```python
from build123d import *

# Parameters (mm, degrees)
F0_R     = 4.677056
F1_DEPTH = 5


with BuildPart() as f1:
    # F0 (on Front) → F1 (new body)
    with BuildSketch(Plane.XZ):
        with BuildLine():
            ThreePointArc((8.500315, 5.267318), (9.510565, 3.09017), (9.972951, 0.73501))
            ThreePointArc((9.972951, 0.73501), (12.080664, 2.122816), (13.312307, 4.325431))
            ThreePointArc((13.312307, 4.325431), (11.021222, 5.383442), (8.500315, 5.267318))
        make_face()
        with BuildLine():
            ThreePointArc((3.780847, 9.25771), (5.877853, 8.09017), (7.636259, 6.456589))
            ThreePointArc((7.636259, 6.456589), (8.525703, 8.81823), (8.227458, 11.324125))
            ThreePointArc((8.227458, 11.324125), (5.752048, 10.833408), (3.780847, 9.25771))
        make_face()
        with BuildLine():
            ThreePointArc((-2.382776, 9.711971), (0, 10), (2.382776, 9.711971))
            ThreePointArc((2.382776, 9.711971), (1.714213, 12.145381), (0, 13.997388))
            ThreePointArc((0, 13.997388), (-1.714213, 12.145381), (-2.382776, 9.711971))
        make_face()
        with BuildLine():
            ThreePointArc((-7.636259, 6.456589), (-5.877853, 8.09017), (-3.780847, 9.25771))
            ThreePointArc((-3.780847, 9.25771), (-5.752048, 10.833408), (-8.227458, 11.324125))
            ThreePointArc((-8.227458, 11.324125), (-8.525703, 8.81823), (-7.636259, 6.456589))
        make_face()
        with BuildLine():
            ThreePointArc((-9.972951, 0.73501), (-9.510565, 3.09017), (-8.500315, 5.267318))
            ThreePointArc((-8.500315, 5.267318), (-11.021222, 5.383442), (-13.312307, 4.325431))
            ThreePointArc((-13.312307, 4.325431), (-12.080664, 2.122816), (-9.972951, 0.73501))
        make_face()
        with BuildLine():
            ThreePointArc((-13.312307, -4.325431), (-11.021222, -5.383442), (-8.500315, -5.267318))
            ThreePointArc((-8.500315, -5.267318), (-9.510565, -3.09017), (-9.972951, -0.73501))
            ThreePointArc((-9.972951, -0.73501), (-12.080664, -2.122816), (-13.312307, -4.325431))
        make_face()
        with BuildLine():
            ThreePointArc((-8.227458, -11.324125), (-5.752048, -10.833408), (-3.780847, -9.25771))
            ThreePointArc((-3.780847, -9.25771), (-5.877853, -8.09017), (-7.636259, -6.456589))
            ThreePointArc((-7.636259, -6.456589), (-8.525703, -8.81823), (-8.227458, -11.324125))
        make_face()
        with BuildLine():
            ThreePointArc((0, -13.997388), (1.714213, -12.145381), (2.382776, -9.711971))
            ThreePointArc((2.382776, -9.711971), (0, -10), (-2.382776, -9.711971))
            ThreePointArc((-2.382776, -9.711971), (-1.714213, -12.145381), (0, -13.997388))
        make_face()
        with BuildLine():
            ThreePointArc((8.227458, -11.324125), (8.525703, -8.81823), (7.636259, -6.456589))
            ThreePointArc((7.636259, -6.456589), (5.877853, -8.09017), (3.780847, -9.25771))
            ThreePointArc((3.780847, -9.25771), (5.752048, -10.833408), (8.227458, -11.324125))
        make_face()
        with BuildLine():
            ThreePointArc((13.312307, -4.325431), (12.080664, -2.122816), (9.972951, -0.73501))
            ThreePointArc((9.972951, -0.73501), (9.510565, -3.09017), (8.500315, -5.267318))
            ThreePointArc((8.500315, -5.267318), (11.021222, -5.383442), (13.312307, -4.325431))
        make_face()
        with BuildLine():
            ThreePointArc((9.972951, -0.73501), (9.993236, -0.367754), (10, 0))
            ThreePointArc((10, 0), (9.993236, 0.367754), (9.972951, 0.73501))
            ThreePointArc((9.972951, 0.73501), (9.510565, 3.09017), (8.500315, 5.267318))
            ThreePointArc((8.500315, 5.267318), (8.09017, 5.877853), (7.636259, 6.456589))
            ThreePointArc((7.636259, 6.456589), (5.877853, 8.09017), (3.780847, 9.25771))
            ThreePointArc((3.780847, 9.25771), (3.09017, 9.510565), (2.382776, 9.711971))
            ThreePointArc((2.382776, 9.711971), (0, 10), (-2.382776, 9.711971))
            ThreePointArc((-2.382776, 9.711971), (-3.09017, 9.510565), (-3.780847, 9.25771))
            ThreePointArc((-3.780847, 9.25771), (-5.877853, 8.09017), (-7.636259, 6.456589))
            ThreePointArc((-7.636259, 6.456589), (-8.09017, 5.877853), (-8.500315, 5.267318))
            ThreePointArc((-8.500315, 5.267318), (-9.510565, 3.09017), (-9.972951, 0.73501))
            ThreePointArc((-9.972951, 0.73501), (-10, 0), (-9.972951, -0.73501))
            ThreePointArc((-9.972951, -0.73501), (-9.510565, -3.09017), (-8.500315, -5.267318))
            ThreePointArc((-8.500315, -5.267318), (-8.09017, -5.877853), (-7.636259, -6.456589))
            ThreePointArc((-7.636259, -6.456589), (-5.877853, -8.09017), (-3.780847, -9.25771))
            ThreePointArc((-3.780847, -9.25771), (-3.09017, -9.510565), (-2.382776, -9.711971))
            ThreePointArc((-2.382776, -9.711971), (0, -10), (2.382776, -9.711971))
            ThreePointArc((2.382776, -9.711971), (3.09017, -9.510565), (3.780847, -9.25771))
            ThreePointArc((3.780847, -9.25771), (5.877853, -8.09017), (7.636259, -6.456589))
            ThreePointArc((7.636259, -6.456589), (8.09017, -5.877853), (8.500315, -5.267318))
            ThreePointArc((8.500315, -5.267318), (9.510565, -3.09017), (9.972951, -0.73501))
        make_face()
        Circle(F0_R, mode=Mode.SUBTRACT)
    extrude(amount=F1_DEPTH)


solid = f1.part
```
Check sheet for the modelled part. Datum: model origin and axes. Units: mm. A direction names the side the tool comes from. Round coordinates to 2 decimals unless told otherwise and drop trailing zeros. Order: outer loops, then holes, each group sorted by start corner. A loop starts at its lowest first (then second) coordinate and runs counter-clockwise, first axis right, second up. Notation, with made-up numbers: M 3,-1 L 33,-1 A12 cw 33,19 Z; hole C 57,42 d1. An arc over 180 degrees is marked long. Answer in a Markdown table with one row per item.
(1) Section check D-D on z = -12. Record the boundary of the cut face in (x, y), plus the area to 3 significant figures.
Findings:
| item | result |
|---|---|
| outline | M -1.79,-5 L 1.79,-5 L 1.79,0 L -1.79,0 Z |
| area | 17.9 mm^2 |
(2) Gauge pin test, flat ends, axial feed: pin 1 (3 mm diameter, centred on y = -1.5, z = -7.5, fed in from +X); pin 2 (8.5 mm diameter, centred on x = 0, z = 0, fed in from -Y); pin 3 (3 mm diameter, centred on y = -4, z = -6, fed in from -X). Record the tip position at first contact, or that the pin passes through.
Findings:
| item | result |
|---|---|
| pin 1 | stops at x = 8.54 |
| pin 2 | passes through |
| pin 3 | stops at x = -13.08 |
(3) Section check B-B on x = -2.75. Record the boundary of the cut face in (y, z).
Findings:
| item | result |
|---|---|
| outline | M -5,-9.61 L 0,-9.61 L 0,-3.78 L -5,-3.78 Z; M -5,3.78 L 0,3.78 L 0,9.61 L -5,9.61 Z |
(4) Material ranges on line 1 along X through (y, z) = (-2.6, 1.75); line 2 along X through (y, z) = (-1.4, 2.5); line 3 along Z through (x, y) = (-0.25, -3.25), recorded low to high. Write a range as from..to.
Findings:
| item | result |
|---|---|
| line 1 | x = -11.7..-4.34, 4.34..11.7 |
| line 2 | x = -12.4..-3.95, 3.95..12.4 |
| line 3 | z = -13.82..-4.67, 4.67..13.82 |
(5) Set-up check for faces 1 (the cylindrical face through (-3.08, -2.465, 9.514)), 2 (the cylindrical face through (4.461, -2.465, 1.405)), 3 (the cylindrical face through (5.72, -2.46, -10.82)): record each of +Z, -Z, +X, -X, +Y, -Y from which the full face is reachable in a straight line by a thin tool's end or side.
Findings:
| item | result |
|---|---|
| face 1 | +Z, +Y, -Y |
| face 2 | +Y, -Y |
| face 3 | -Z, +Y, -Y |
(6) Section check C-C on z = 10.25. Record the boundary of the cut face in (x, y).
Findings:
| item | result |
|---|---|
| outline | M -8.51,-5 L -4.78,-5 L -4.78,0 L -8.51,0 Z; M -2.34,-5 L 2.34,-5 L 2.34,0 L -2.34,0 Z; M 4.78,-5 L 8.51,-5 L 8.51,0 L 4.78,0 Z |
(7) Draft check along Z on faces 4 (the flat face through (6, 0, 0)), 5 (the cylindrical face through (12.105, -2.465, -2.149)), 6 (the cylindrical face through (-10, -2, 0)), 7 (the cylindrical face through (-1.697, -2.465, 12.176)). Enter one of: +Z half, -Z half, draft (parallel to the pull), parting line (faces both ways), or undercut.
Findings:
| item | result |
|---|---|
| face 4 | draft |
| face 5 | undercut |
| face 6 | undercut |
| face 7 | +Z half |
